```python
from build123d import *

# Parameters (mm, degrees)
SKETCH1_W                = 127
SKETCH1_H                = 76.2
BOSS_EXTRUDE1_DEPTH      = 5.08
CUT_EXTRUDE1_REACH       = 7.08
SKETCH2_W                = 25.4
SKETCH2_H                = 5.08
SKETCH3_W                = 25.4
SKETCH3_H                = 5.08
CUT_EXTRUDE2_DEPTH       = 6.08
CUT_EXTRUDE3_REACH       = 7.08
SKETCH4_R                = 6
SKETCH8_W                = 3.599999912
SKETCH8_H                = 7.62
CUT_EXTRUDE6_DEPTH       = 5.08
SKETCH9_W                = 5.4483
SKETCH9_H                = 2.3241
CUT_EXTRUDE7_DEPTH       = 5.08
M3_CLEARANCE_HOLE1_D     = 3.6
M3_CLEARANCE_HOLE1_DEPTH = 5.08


with BuildPart() as part:
    # Sketch1 → Boss-Extrude1 (new body)
    with BuildSketch(Plane.XY):
        with Locations((63.5, 38.1)):
            Rectangle(SKETCH1_W, SKETCH1_H)
    extrude(amount=BOSS_EXTRUDE1_DEPTH)

    # Sketch2 → Cut-Extrude1 (cut, up to next)
    with BuildSketch(Plane.XY.offset(5.08), mode=Mode.PRIVATE) as cut_extrude1_sk1:
        with Locations((25.4, 2.54)):
            Rectangle(SKETCH2_W, SKETCH2_H)
    cut_extrude1_tool1 = extrude(cut_extrude1_sk1.sketch, amount=-CUT_EXTRUDE1_REACH, mode=Mode.PRIVATE) & part.part
    add(cut_extrude1_tool1.solids().sort_by_distance((25.4, 2.54, 5.08))[0], mode=Mode.SUBTRACT)
    # Sketch2 → Cut-Extrude1 (cut, up to next)
    with BuildSketch(Plane.XY.offset(5.08), mode=Mode.PRIVATE) as cut_extrude1_sk2:
        with Locations((101.6, 2.54)):
            Rectangle(SKETCH2_W, SKETCH2_H)
    cut_extrude1_tool2 = extrude(cut_extrude1_sk2.sketch, amount=-CUT_EXTRUDE1_REACH, mode=Mode.PRIVATE) & part.part
    add(cut_extrude1_tool2.solids().sort_by_distance((101.6, 2.54, 5.08))[0], mode=Mode.SUBTRACT)

    # Sketch3 → Cut-Extrude2 (cut, through all)
    with BuildSketch(Plane.XY.offset(5.08)):
        with Locations((25.4, 73.66)):
            Rectangle(SKETCH3_W, SKETCH3_H)
        with Locations((101.6, 73.66)):
            Rectangle(SKETCH3_W, SKETCH3_H)
    extrude(amount=-CUT_EXTRUDE2_DEPTH, mode=Mode.SUBTRACT)

    # Sketch4 → Cut-Extrude3 (cut, up to next)
    with BuildSketch(Plane.XY.offset(5.08), mode=Mode.PRIVATE) as cut_extrude3_sk1:
        with Locations((63.5, 21.08)):
            Circle(SKETCH4_R)
    cut_extrude3_tool1 = extrude(cut_extrude3_sk1.sketch, amount=-CUT_EXTRUDE3_REACH, mode=Mode.PRIVATE) & part.part
    add(cut_extrude3_tool1.solids().sort_by_distance((63.5, 21.08, 5.08))[0], mode=Mode.SUBTRACT)

    # Sketch8 → Cut-Extrude6 (cut)
    with BuildSketch(Plane.XY.offset(5.08)):
        with Locations((17.039999956, 8.89)):
            Rectangle(SKETCH8_W, SKETCH8_H)
    cut_extrude6 = extrude(amount=-CUT_EXTRUDE6_DEPTH, mode=Mode.SUBTRACT)

    # Sketch9 → Cut-Extrude7 (cut)
    with BuildSketch(Plane.XY.offset(5.08)):
        with Locations((17.039999956, 8.89)):
            Rectangle(SKETCH9_W, SKETCH9_H)
    cut_extrude7 = extrude(amount=-CUT_EXTRUDE7_DEPTH, mode=Mode.SUBTRACT)

    # Mirror1: Cut-Extrude6, Cut-Extrude7 across plane
    add(cut_extrude6.mirror(Plane.ZY.offset(-63.5)), mode=Mode.SUBTRACT)
    add(cut_extrude7.mirror(Plane.ZY.offset(-63.5)), mode=Mode.SUBTRACT)

    # M3 Clearance Hole1
    with Locations(Plane.XY.offset(5.08)):
        with Locations((39.5, 30.08), (72.5, 30.08), (72.5, 12.08), (39.5, 12.08)):
            Hole(M3_CLEARANCE_HOLE1_D / 2, depth=M3_CLEARANCE_HOLE1_DEPTH)


solid = part.part
```
The model under review builds one solid part; all positions refer to its coordinate system, in mm. A direction names the side the tool comes from. Round coordinates to 2 decimals unless told otherwise and drop trailing zeros. Loops run counter-clockwise (first coordinate to the right, second up) from the corner with the lowest first, then second, coordinate; pieces in that order, holes last. Notation, with made-up numbers: (26.5, 17.5) - (43.5, 17.5) arc R29 cw to (43.5, 45.5) - close; hole circle Ø11 at (23.25, 88.5). An arc over 180 degrees is marked (long way). Write each question's results on one line, items separated by ' | '. Start each with the question number.
Q1. Take a section at D-D on z = 1.8. Give the number of separate pieces and of enclosed holes in the cut face, plus the area to 3 significant figures.
Q2. Tool access review of faces 1 (the flat face through (6, 76.2, 3)), 2 (the flat face through (107.236, 9, 3)), 3 (the flat face through (108.16, 11, 3)), 4 (the flat face through (38.1, 74, 3)): name each direction out of +Z, -Z, +X, -X, +Y, -Y from which nothing blocks a thin tool from reaching the whole face with its end or side.
Q3. Draft analysis for pull direction Y (two halves, no side actions). For faces 5 (the flat face through (25, 71.12, 3)), 6 (the flat face through (12.7, 3, 3)), 7 (the flat face through (14.316, 9, 3)), state which applies: pulls with the +Y half, pulls with the -Y half, needs draft (parallel to the pull), parting line crosses it, or undercut.
Q4. Insertion check: P1, Ø2, axis at x = 17.5, z = 4.5, coming from the -Y side; P2, Ø0.5, axis at x = 112, z = 3, coming from the -Y side. Each pin has a flat end and moves straight along its axis. Give the tip position at first contact, or say it passes through.
Q5. Wall thickness on line 1 along Y through (x, z) = (72.5, 2.55); line 2 along X through (y, z) = (8.5, 0.5); line 3 along X through (y, z) = (72.5, 3.65): over which ranges is each line inside the solid? List them lowest first. Write a range as [from, to].
Q6. Take a section at A-A on x = 72.5. Give the boundary of the cut face in (y, z), plus the area to 3 significant figures.
Q7. Take a section at B-B on y = 30.08. Give the boundary of the cut face in (x, z), plus the area to 3 significant figures.
Q8. Take a section at C-C on x = 96.5. Give the boundary of the cut face in (y, z), plus the area to 3 significant figures.
Data:
1) separate pieces: 1 | enclosed holes: 5 | area: 8,940 mm²
2) face 1: +Z, -Z, +X, -X, +Y | face 2: +Z, -Z | face 3: +Z, -Z, -Y | face 4: +Z, -Z, +Y
3) face 5: pulls with the +Y half | face 6: needs draft | face 7: undercut
4) P1: stops at y = 12.7 | P2: stops at y = 5.08
5) line 1: y = [0, 10.28], [13.88, 28.28], [31.88, 76.2] | line 2: x = [0, 14.32], [19.76, 107.24], [112.68, 127] | line 3: x = [0, 12.7], [38.1, 88.9], [114.3, 127]
6) outline: (0, 0) - (10.28, 0) - (10.28, 5.08) - (0, 5.08) - close; (13.88, 0) - (28.28, 0) - (28.28, 5.08) - (13.88, 5.08) - close; (31.88, 0) - (76.2, 0) - (76.2, 5.08) - (31.88, 5.08) - close | area: 351 mm²
7) outline: (0, 0) - (37.7, 0) - (37.7, 5.08) - (0, 5.08) - close; (41.3, 0) - (70.7, 0) - (70.7, 5.08) - (41.3, 5.08) - close; (74.3, 0) - (127, 0) - (127, 5.08) - (74.3, 5.08) - close | area: 609 mm²
8) outline: (5.08, 0) - (71.12, 0) - (71.12, 5.08) - (5.08, 5.08) - close | area: 335 mm²
